from build123d import *

# Parameters (mm, degrees)
CROQUIS1_R                          = 26
SALIENTE_EXTRUIR1_DEPTH             = 6.5
CROQUIS2_R                          = 20
CROQUIS2_R_2                        = 18
SALIENTE_EXTRUIR3_DEPTH             = 0.2
SALIENTE_EXTRUIR4_START             = 0.2
CROQUIS4_R                          = 20
CROQUIS4_R_2                        = 18
SALIENTE_EXTRUIR4_DEPTH             = 0.2
CROQUIS5_R                          = 18
CORTAR_EXTRUIR1_DEPTH               = 5
CORTAR_EXTRUIR2_START               = -5
CROQUIS6_R                          = 18
CORTAR_EXTRUIR2_DEPTH               = 5
SALIENTE_EXTRUIR5_REACH             = 39.673
CROQUIS7_R                          = 6.5
CROQUIS7_R_2                        = 4.05
SALIENTE_EXTRUIR5_DIRECTION_2_REACH = 39.673
CROQUIS8_R                          = 4.05
CORTAR_EXTRUIR3_DEPTH               = 39


with BuildPart() as part:
    # Croquis1 → Saliente-Extruir1 (new, symmetric)
    with BuildSketch(Plane.XY):
        with Locations(Location((0, 0, 0), (0, 0, 180))):
            Circle(CROQUIS1_R)
    extrude(amount=SALIENTE_EXTRUIR1_DEPTH, both=True)

    # Croquis2 → Saliente-Extruir3 (add)
    with BuildSketch(Plane.XY.offset(6.5)):
        Circle(CROQUIS2_R)
        Circle(CROQUIS2_R_2, mode=Mode.SUBTRACT)
    extrude(amount=SALIENTE_EXTRUIR3_DEPTH)

    # Croquis4 → Saliente-Extruir4 (add)
    with BuildSketch(Plane(origin=(0, 0, -6.5), x_dir=(-1, 0, 0), z_dir=(0, 0, -1)).offset(SALIENTE_EXTRUIR4_START)):
        with Locations(Location((0, 0, 0), (0, 0, 180))):
            Circle(CROQUIS4_R)
        with Locations(Location((0, 0, 0), (0, 0, 180))):
            Circle(CROQUIS4_R_2, mode=Mode.SUBTRACT)
    extrude(amount=-SALIENTE_EXTRUIR4_DEPTH)

    # Croquis5 → Cortar-Extruir1 (cut)
    with BuildSketch(Plane(origin=(0, 0, -6.5), x_dir=(-1, 0, 0), z_dir=(0, 0, -1))):
        with Locations(Location((0, 0, 0), (0, 0, 180))):
            Circle(CROQUIS5_R)
    extrude(amount=-CORTAR_EXTRUIR1_DEPTH, mode=Mode.SUBTRACT)

    # Croquis6 → Cortar-Extruir2 (cut)
    with BuildSketch(Plane.XY.offset(6.5).offset(CORTAR_EXTRUIR2_START)):
        Circle(CROQUIS6_R)
    extrude(amount=CORTAR_EXTRUIR2_DEPTH, mode=Mode.SUBTRACT)

    # Saliente-Extruir5: up to this face of the body (flat: up to its plane)
    saliente_extruir5_end = Plane(part.part.faces().sort_by_distance((-19.434314575, 0, -6.7))[0])
    # Croquis7 → Saliente-Extruir5 (add, up to the picked face)
    with BuildSketch(Plane(origin=(0, 0, -1.5), x_dir=(-1, 0, 0), z_dir=(0, 0, -1)), mode=Mode.PRIVATE) as saliente_extruir5_sk1:
        with Locations(Location((0, 0, 0), (0, 0, 180))):
            Circle(CROQUIS7_R)
        with Locations(Location((0, 0, 0), (0, 0, 180))):
            Circle(CROQUIS7_R_2, mode=Mode.SUBTRACT)
    saliente_extruir5_tool1 = split(extrude(saliente_extruir5_sk1.sketch, amount=SALIENTE_EXTRUIR5_REACH, mode=Mode.PRIVATE), bisect_by=saliente_extruir5_end, keep=Keep.BOTH, mode=Mode.PRIVATE)
    add(saliente_extruir5_tool1.solids().sort_by(Axis((-6.316152, 0, -1.5), (0, 0, -1)))[0])

    # Saliente-Extruir5 direction 2: up to this face of the body (flat: up to its plane)
    saliente_extruir5_direction_2_end = Plane(part.part.faces().sort_by_distance((-19.434314575, 0, 6.7))[0])
    # Croquis7 → Saliente-Extruir5 direction 2 (add, up to the picked face)
    with BuildSketch(Plane(origin=(0, 0, -1.5), x_dir=(-1, 0, 0), z_dir=(0, 0, -1)), mode=Mode.PRIVATE) as saliente_extruir5_direction_2_sk1:
        with Locations(Location((0, 0, 0), (0, 0, 180))):
            Circle(CROQUIS7_R)
        with Locations(Location((0, 0, 0), (0, 0, 180))):
            Circle(CROQUIS7_R_2, mode=Mode.SUBTRACT)
    saliente_extruir5_direction_2_tool1 = split(extrude(saliente_extruir5_direction_2_sk1.sketch, amount=-SALIENTE_EXTRUIR5_DIRECTION_2_REACH, mode=Mode.PRIVATE), bisect_by=saliente_extruir5_direction_2_end, keep=Keep.BOTH, mode=Mode.PRIVATE)
    add(saliente_extruir5_direction_2_tool1.solids().sort_by(Axis((-6.316152, 0, -1.5), (0, 0, 1)))[0])

    # Croquis8 → Cortar-Extruir3 (cut, symmetric)
    with BuildSketch(Plane(origin=(0, 0, -1.5), x_dir=(-1, 0, 0), z_dir=(0, 0, -1))):
        with Locations(Location((0, 0, 0), (0, 0, 180))):
            Circle(CROQUIS8_R)
    extrude(amount=CORTAR_EXTRUIR3_DEPTH, both=True, mode=Mode.SUBTRACT)


solid = part.part
Geometry check sheet. Reference: the model listing, model coordinates, mm. A direction names the side the tool comes from. Round coordinates to 2 decimals unless told otherwise and drop trailing zeros. Write each loop counter-clockwise with the first axis right and the second up, starting at its lowest first coordinate (ties: lowest second). Pieces come first, ordered by that corner, then holes. Notation, with made-up numbers: (-2.75, 28.5) -> (26.25, 28.5) arc R11 cw to (26.25, 43.5) -> close; hole circle Ø11 at (23.25, 79.5). An arc over 180 degrees is marked (long way). One line per item, written item: value. Start each with the question number.
(1) Access from +Z, -Z, +X, -X, +Y, -Y to the whole of each face (thin tool, end or side, straight path). Record for faces 4 (the flat face through (0, -8, 1.5)), 5 (the cylindrical face through (-13.267, -12.165, -4.136)), 6 (the flat face through (3, 3, 6.7)).
(2) Go/stop test with flat-tipped pins: pin 1 Ø6 at (x, z) = (6, 3.5) entering from +Y; pin 2 Ø4 at (x, z) = (-1, 0.5) entering from +Y; pin 3 Ø3 at (y, z) = (19.5, 5) entering from -X. Record where each tip stops, or that it passes through.
(3) Scan lines: line 1 (Y direction, x = 0, z = 2.85); line 2 (Z direction, x = 20, y = 1.5); line 3 (X direction, y = -3.5, z = -5.5). Record each from-to range of solid material in increasing order. Write a range as [from, to].
(4) Draft check along Y on faces 1 (the flat face through (-13.4, 15.3, -6.5)), 2 (the cylindrical face through (20.633, 15.821, 0.091)), 3 (the cylindrical face through (-0.878, 3.954, -0.094)). Enter one of: +Y half, -Y half, draft (parallel to the pull), parting line (faces both ways), or undercut.
(5) Cross-section at D-D, the plane z = 0. Record the cut outline in (x, y).
(6) Cross-section at A-A, the plane z = -3.25. Record the cut outline in (x, y), and give its area (3 significant figures).
Answer:
1. face 4: +Z
1. face 5: -Z
1. face 6: +Z, +X, -X, +Y, -Y
2. pin 1: y = 25.83
2. pin 2: y = 26
2. pin 3: x = -18.76
3. line 1: [-26, -18], [-6.5, -4.05], [4.05, 6.5], [18, 26]
3. line 2: [-6.5, 6.5]
3. line 3: [-25.76, -17.66], [-5.48, -2.04], [2.04, 5.48], [17.66, 25.76]
4. face 1: draft
4. face 2: parting line
4. face 3: undercut
5. outline: circle Ø52 at (0, 0); hole circle Ø8.1 at (0, 0)
6. outline: circle Ø52 at (0, 0); circle Ø13 at (0, 0); hole circle Ø36 at (0, 0); hole circle Ø8.1 at (0, 0)
6. area: 1,190 mm²
